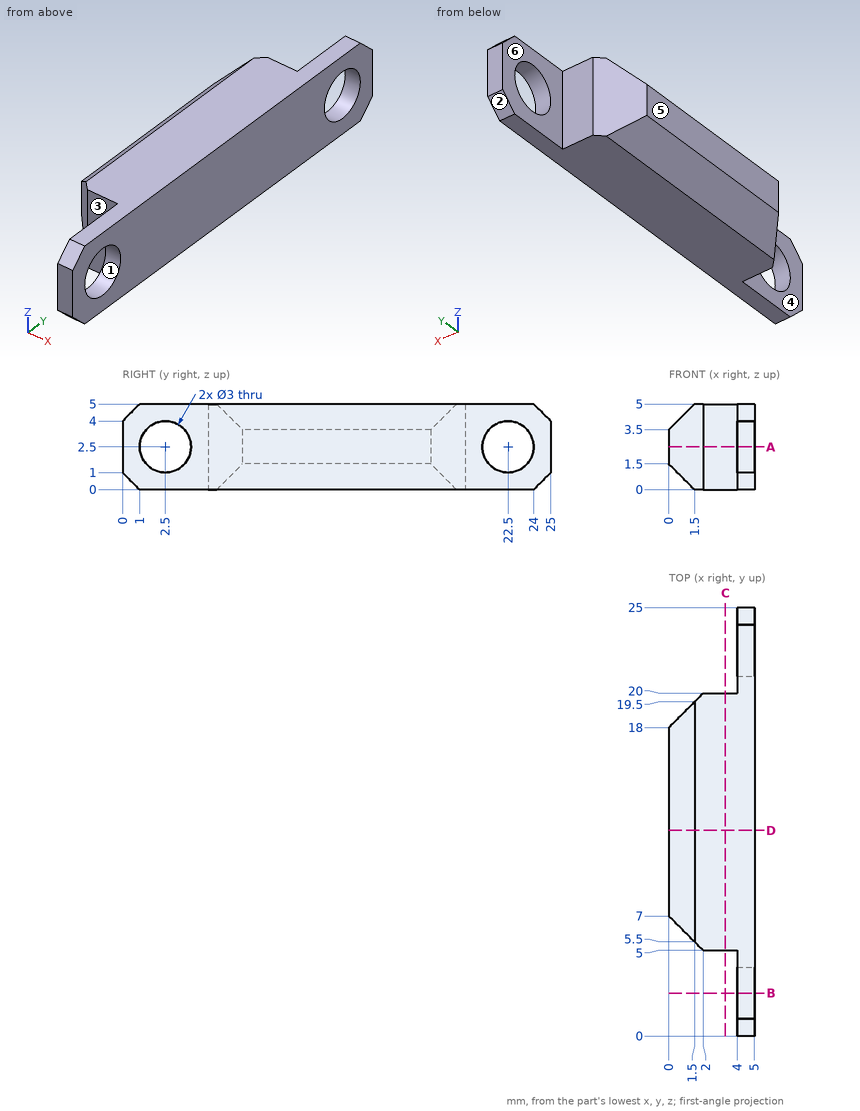
The figure shows three views and two pictorial views of one solid part (mm, origin at its lowest corner). Answer the questions. A direction names the side the tool comes from. Coordinates: 2 decimals unless noted, no trailing zeros. Write each loop counter-clockwise with the first axis right and the second up, starting at its lowest first coordinate (ties: lowest second). Pieces come first, ordered by that corner, then holes.
1. Flat-ended cylindrical pins translate along their axes: pin 1 (1.8 mm diameter, centred on y = 2.5, z = 2.5, fed in from +X); pin 2 (2 mm diameter, centred on x = 2.5, z = 3.5, fed in from +Y); pin 3 (2 mm diameter, centred on x = 2.5, z = 3, fed in from -Y); pin 4 (2.5 mm diameter, centred on y = 2, z = 2, fed in from -X). Find the tip coordinate at first contact, or state that the pin passes through.
Results list:
pin 1: passes through
pin 2: stops at y = 20
pin 3: stops at y = 5
pin 4: stops at x = 4
2. Consider line 1 along Y through (x, z) = (4.75, 2.5); line 2 along Z through (x, y) = (4.45, 2.5); line 3 along Y through (x, z) = (3.85, 2.45). Determine where each line is inside the solid, lowest interval first.
Results list:
line 1: y = 0 to 1, 4 to 21, 24 to 25
line 2: z = 0 to 1, 4 to 5
line 3: y = 5 to 20
3. For the marked faces 4, 5 and 6, determine the directions among +Z, -Z, +X, -X, +Y, -Y from which every point of the face is accessible in a straight line to the end or side of a thin tool.
Results list:
face 4: +Z, -Z, -X, -Y
face 5: +Z, -Z, -X, +Y, -Y
face 6: +Z, -Z, -X, +Y
4. The part is cut by section D-D, the plane y = 12. Write down the section's boundary in (x, z), and give its area (4 significant figures).
Results list:
outline: (0, 1.5) - (1.5, 0) - (5, 0) - (5, 5) - (1.5, 5) - (0, 3.5) - close
area: 22.75 mm2
5. The part is cut by section A-A, the plane z = 2.5. Write down the section's boundary in (x, y), and give its area (3 significant figures).
Results list:
outline: (0, 7) - (2, 5) - (4, 5) - (4, 4) - (5, 4) - (5, 21) - (4, 21) - (4, 20) - (2, 20) - (0, 18) - close; (4, 0) - (5, 0) - (5, 1) - (4, 1) - close; (4, 24) - (5, 24) - (5, 25) - (4, 25) - close
area: 75.0 mm2
6. The part is cut by section C-C, the plane x = 3.3. Write down the section's boundary in (y, z).
Results list:
outline: (5, 0) - (20, 0) - (20, 5) - (5, 5) - close
7. The part is cut by section B-B, the plane y = 2.5. Write down the section's boundary in (x, z), and give its area (3 significant figures).
Results list:
outline: (4, 0) - (5, 0) - (5, 1) - (4, 1) - close; (4, 4) - (5, 4) - (5, 5) - (4, 5) - close
area: 2.00 mm2
8. For a pull along Z with two mould halves and no side action, classify the marked faces 1, 2 and 3 as +Z half, -Z half, draft (parallel to the pull), parting line (faces both ways), or undercut.
Results list:
face 1: undercut
face 2: -Z half
face 3: draft
